Check sheet for the modelled part. Datum: model origin and axes. Units: mm. Face numbers are marked on the shaded views. A direction names the side the tool comes from. Give positions to 0.01 mm unless a question says otherwise; leave off trailing zeros. Loops run counter-clockwise (first coordinate to the right, second up) from the corner with the lowest first, then second, coordinate; pieces in that order, holes last.
```python
from build123d import *

# Parameters (mm, degrees)
SKETCH_1_R               = 10
SKETCH_1_R_2             = 3.15
EXTRUDE_1_DEPTH          = 30
CUT_EXTRUDE_1_DEPTH      = 34.166247904
CUT_EXTRUDE_1_DEPTH_BACK = 34.166247904
SKETCH_2_R               = 1.5
SKETCH_3_R               = 1.5
CUT_EXTRUDE_2_DEPTH      = 34.166248063
SKETCH_4_R               = 6.15
CUT_EXTRUDE_3_DEPTH      = 18
CUT_EXTRUDE_START        = -10
SKETCH_5_R               = 3
CUT_EXTRUDE_4_DEPTH      = 3


with BuildPart() as part:
    # 草图1 → 凸台-拉伸1 (new body)
    with BuildSketch(Plane(origin=(0, 0, 0), x_dir=(1, 0, 0), z_dir=(0, 1, 0))):
        with Locations(Location((0, 0, 0), (0, 0, 270))):
            Circle(SKETCH_1_R)
        with Locations(Location((0, 0, 0), (0, 0, 270))):
            Circle(SKETCH_1_R_2, mode=Mode.SUBTRACT)
    extrude(amount=EXTRUDE_1_DEPTH)

    # 草图2 → 切除-拉伸1 (cut, two sides: drawn at the far end of the back side and taken through both)
    with BuildSketch(Plane(origin=(0, 0, 0), x_dir=(0, 0, -1), z_dir=(1, 0, 0)).offset(-CUT_EXTRUDE_1_DEPTH_BACK)):
        with Locations((0, 7)):
            Circle(SKETCH_2_R)
    extrude(amount=CUT_EXTRUDE_1_DEPTH + CUT_EXTRUDE_1_DEPTH_BACK, mode=Mode.SUBTRACT)

    # 草图3 → 切除-拉伸2 (cut, through all)
    with BuildSketch(Plane.XY):
        with Locations(Location((0, 24, 0), (0, 0, 90))):
            Circle(SKETCH_3_R)
    extrude(amount=-CUT_EXTRUDE_2_DEPTH, mode=Mode.SUBTRACT)

    # 草图4 → 切除-拉伸3 (cut)
    with BuildSketch(Plane.XZ):
        with Locations(Location((0, 0, 0), (0, 0, 270))):
            Circle(SKETCH_4_R)
    extrude(amount=-CUT_EXTRUDE_3_DEPTH, mode=Mode.SUBTRACT)

    # 草图5 → 切除-拉伸4 (cut)
    with BuildSketch(Plane.XY.offset(CUT_EXTRUDE_START)):
        with Locations(Location((0, 24, 0), (0, 0, 90))):
            Circle(SKETCH_5_R)
    extrude(amount=CUT_EXTRUDE_4_DEPTH, mode=Mode.SUBTRACT)


solid = part.part
```
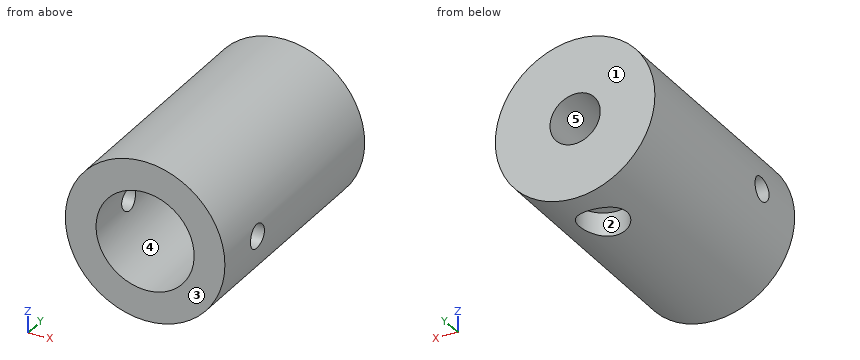
(1) Access from +Z, -Z, +X, -X, +Y, -Y to the whole of each face (thin tool, end or side, straight path). Record for the marked faces 4 and 5.
(2) Material ranges on line 1 (Y direction, x = 8.05, z = 0); line 2 (Y direction, x = -3.5, z = 1); line 3 (X direction, y = 22.5, z = -7.5), recorded low to high.
(3) Section check B-B on y = 7. Record the boundary of the cut face in (x, z).
(4) Release check for a two-part mould opening along Y. For the marked faces 1, 2 and 3 record: pulls with the +Y half, pulls with the -Y half, needs draft (parallel to the pull), parting line crosses it, or undercut.
(5) Section check C-C on y = 18.5. Record the boundary of the cut face in (x, z).
(6) Section check D-D on x = -7. Record the boundary of the cut face in (y, z), plus the area to 3 significant figures.
(7) Gauge pin test, flat ends, axial feed: pin 1 Ø1 at (y, z) = (9.5, 3.5) entering from +X; pin 2 Ø4 at (x, z) = (-6.5, -1.5) entering from -Y; pin 3 Ø3 at (y, z) = (10, -4.5) entering from -X; pin 4 Ø6 at (x, y) = (7, 9) entering from -Z. Record the tip position at first contact, or that the pin passes through.
(8) Section check A-A on x = 0. Record the boundary of the cut face in (y, z), plus the area to 3 significant figures.
Computed values:
1. face 4: -Y
1. face 5: +Y, -Y
2. line 1: y = 0 to 5.5, 8.5 to 30
2. line 2: y = 18 to 30
2. line 3: x = -6.61 to -2.6, 2.6 to 6.61
3. outline: (-9.89, -1.5) arc R10 ccw to (9.89, -1.5) - (5.96, -1.5) arc R6.15 cw to (-5.96, -1.5) - close; (-9.89, 1.5) - (-5.96, 1.5) arc R6.15 cw to (5.96, 1.5) - (9.89, 1.5) arc R10 ccw to start
4. face 1: pulls with the +Y half
4. face 2: undercut
4. face 3: pulls with the -Y half
5. outline: circle Ø20 at (0, 0); hole circle Ø6.3 at (0, 0)
6. outline: (0, -7.14) - (30, -7.14) - (30, 7.14) - (0, 7.14) - close; hole circle Ø3 at (7, 0)
6. area: 421 mm2
7. pin 1: stops at x = 9.54
7. pin 2: stops at y = 0
7. pin 3: stops at x = -9.54
7. pin 4: stops at z = -9.17
8. outline: (0, -10) - (21, -10) - (21, -7) - (22.5, -7) - (22.5, -3.15) - (18, -3.15) - (18, -6.15) - (0, -6.15) - close; (0, 6.15) - (18, 6.15) - (18, 3.15) - (30, 3.15) - (30, 10) - (0, 10) - close; (25.5, -7) - (27, -7) - (27, -10) - (30, -10) - (30, -3.15) - (25.5, -3.15) - close
8. area: 273 mm2
